Could you check a few things on this drawing? It's one solid part, dimensions in mm from its lowest x, y, z. Round coordinates to 2 decimals unless told otherwise and drop trailing zeros. Order: outer loops, then holes, each group sorted by start corner. A loop starts at its lowest first (then second) coordinate and runs counter-clockwise, first axis right, second up.
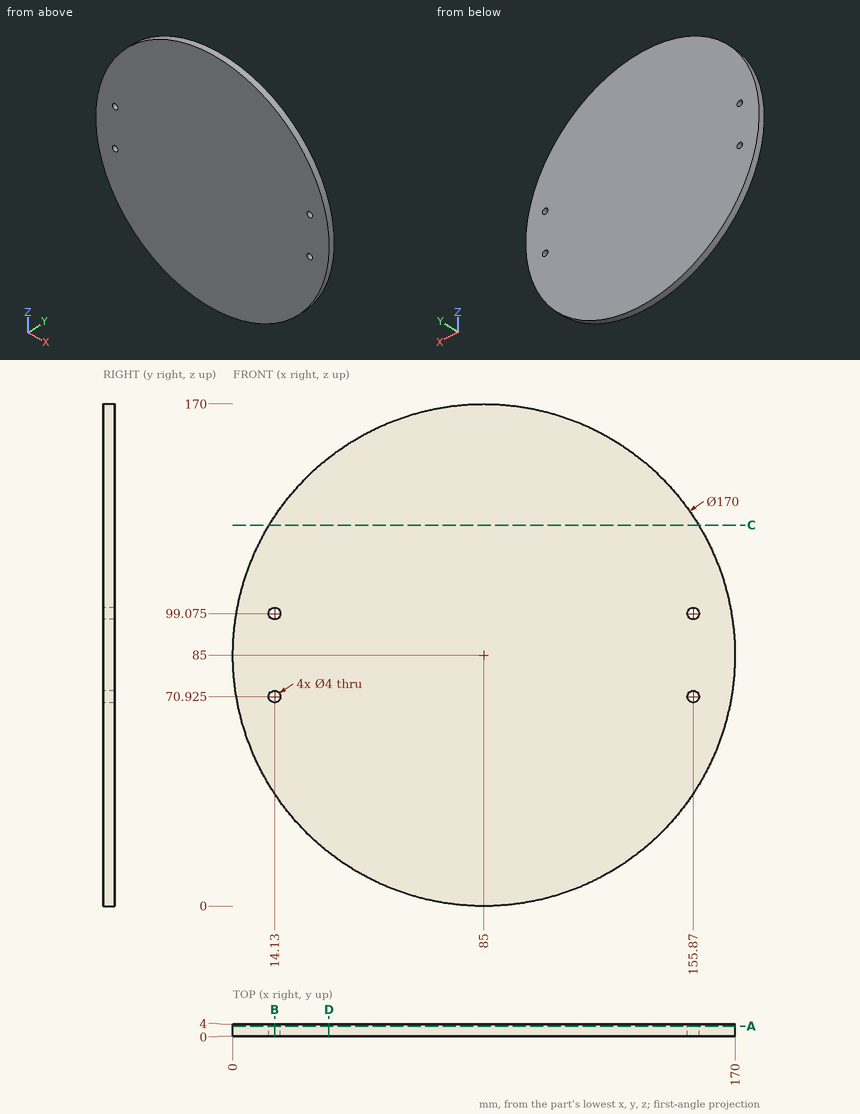
(1) I want a section at D-D, the plane x = 32.5. List the corners of the cut face in (y, z) for me, plus the area to 3 significant figures.
(2) I want a section at A-A, the plane y = 3.35. List the corners of the cut face in (x, z) for me (3 decimals).
(3) I want a section at C-C, the plane z = 129. List the corners of the cut face in (x, y) for me, plus the area to 3 significant figures.
(4) Please list where these lines run through material, in increasing order: probe 1 along Z at (x, y) = (155.87, 1.3) (3 decimals); probe 2 along X at (y, z) = (2.6, 72); probe 3 along X at (y, z) = (0.9, 85.5).
(5) I'm going to push flat-ended pins straight in: pin 1 Ø3 at (x, z) = (155.87, 99.075) entering from +Y; pin 2 Ø2 at (y, z) = (2, 108.5) entering from -X; pin 3 Ø1 at (x, y) = (27, 3) entering from -Z. Where does each tip first touch, or does it pass through?
(6) I want a section at B-B, the plane x = 14.13. List the corners of the cut face in (y, z) for me (3 decimals), plus the area to 3 significant figures.
Ans:
1. outline: (0, 18.15) - (4, 18.15) - (4, 151.85) - (0, 151.85) - close
1. area: 535 mm2
2. outline: circle Ø170 at (85, 85); hole circle Ø4 at (14.13, 70.925); hole circle Ø4 at (14.13, 99.075); hole circle Ø4 at (155.87, 70.925); hole circle Ø4 at (155.87, 99.075)
3. outline: (12.27, 0) - (157.73, 0) - (157.73, 4) - (12.27, 4) - close
3. area: 582 mm2
4. probe 1: z = 38.07 to 68.925, 72.925 to 97.075, 101.075 to 131.93
4. probe 2: x = 1 to 12.44, 15.82 to 154.18, 157.56 to 169
4. probe 3: x = 0 to 170
5. pin 1: passes through
5. pin 2: stops at x = 3.03
5. pin 3: stops at z = 22.4
6. outline: (0, 38.07) - (4, 38.07) - (4, 68.925) - (0, 68.925) - close; (0, 72.925) - (4, 72.925) - (4, 97.075) - (0, 97.075) - close; (0, 101.075) - (4, 101.075) - (4, 131.93) - (0, 131.93) - close
6. area: 343 mm2
